For this review, take the finished solid that the model builds, in its own axes (mm). Face numbers are marked on the shaded views. Round coordinates to 2 decimals unless told otherwise and drop trailing zeros. Loops run counter-clockwise (first coordinate to the right, second up) from the corner with the lowest first, then second, coordinate; pieces in that order, holes last. Notation, with made-up numbers: M 18,0 L 49,0 A24 cw 49,31 Z; hole C 89,76.25 d8. An arc over 180 degrees is marked long. One line per question, with ' | ' between items. Start each with the question number.
1) We need section B-B (y = 0). Give the boundary of the cut face in (x, z).
2) For pin 1 Ø2.5 at (x, z) = (11, -0.5) entering from -Y (3 decimals); pin 2 Ø2 at (x, y) = (12, 9.5) entering from -Z; pin 3 Ø0.5 at (x, y) = (12.5, 5.5) entering from -Z, all flat-tipped, find the tip position at first contact; note any pin that passes through.
3) We need section A-A (z = 0). Give the boundary of the cut face in (x, y).
4) Mouldability with a two-part tool opening along Z and no side actions: class the marked faces 1, 2 and 3 as pulls with the +Z half, pulls with the -Z half, needs draft (parallel to the pull), parting line crosses it, or undercut.
5) For probe 1 along X at (y, z) = (-8.5, -6.75); probe 2 along Z at (x, y) = (14, 0); probe 3 along Z at (x, y) = (12.25, 9.25), list the stretches that pass through material, from the lowest coordinate up. Write a range as from..to.
```python
from build123d import *

# Parameters (mm, degrees)
SCHIZZO5_R                    = 0.75
TAGLIO_ESTRUSIONE1_DEPTH      = 7
TAGLIO_ESTRUSIONE2_REACH      = 26.782
TAGLIO_ESTRUSIONE2_END_RADIUS = 8
SCHIZZO6_R                    = 1.5
TAGLIO_ESTRUSIONE3_REACH      = 26.782
TAGLIO_ESTRUSIONE3_END_RADIUS = 8
SCHIZZO7_R                    = 1.5
SMUSSO1_SIZE                  = 0.5
SMUSSO2_SIZE                  = 0.25
SCHIZZO8_R                    = 5
TAGLIO_ESTRUSIONE4_DEPTH      = 25.781545622
TAGLIO_ESTRUSIONE5_START      = -7
SCHIZZO9_R                    = 8
TAGLIO_ESTRUSIONE5_DEPTH      = 7
TAGLIO_ESTRUSIONE6_DEPTH      = 30.654470544
TAGLIO_ESTRUSIONE6_DEPTH_BACK = 7
SCHIZZO10_W                   = 3
SCHIZZO10_H                   = 1.630303993


with BuildPart() as part:
    # Schizzo4 → Rivoluzione1 (revolve)
    with BuildSketch(Plane.XY, mode=Mode.PRIVATE) as rivoluzione1_sk:
        Polygon((0, 2.5), (0, 8), (7, 8), (7, 12.75), (7.75, 12.75), (8.5, 11.450961894), (8.5, 11.25), (15.5, 11.25), (15.5, 11.450961894), (16.25, 12.75), (17, 12.75), (17, 2.5), align=None)
    revolve(rivoluzione1_sk.sketch.rotate(Axis((0, 0, 0), (1, 0, 0)), 90), axis=Axis((0, 0, 0), (1, 0, 0)))

    # Schizzo5 → Taglio-Estrusione1 (cut)
    with BuildSketch(Plane(origin=(8.5, 0, 0), x_dir=(0, 0, -1), z_dir=(1, 0, 0))):
        with Locations((0, 11.25)):
            Circle(SCHIZZO5_R)
        with Locations((1.953541999, 11.079087221)):
            Circle(SCHIZZO5_R)
        with Locations((3.847726612, 10.571541984)):
            Circle(SCHIZZO5_R)
        with Locations((5.625, 9.742785793)):
            Circle(SCHIZZO5_R)
        with Locations((7.231360609, 8.617999985)):
            Circle(SCHIZZO5_R)
        with Locations((8.617999985, 7.231360609)):
            Circle(SCHIZZO5_R)
        with Locations((9.742785793, 5.625)):
            Circle(SCHIZZO5_R)
        with Locations((10.571541984, 3.847726612)):
            Circle(SCHIZZO5_R)
        with Locations((11.079087221, 1.953541999)):
            Circle(SCHIZZO5_R)
        with Locations((11.25, 0)):
            Circle(SCHIZZO5_R)
        with Locations((11.079087221, -1.953541999)):
            Circle(SCHIZZO5_R)
        with Locations((10.571541984, -3.847726612)):
            Circle(SCHIZZO5_R)
        with Locations((9.742785793, -5.625)):
            Circle(SCHIZZO5_R)
        with Locations((8.617999985, -7.231360609)):
            Circle(SCHIZZO5_R)
        with Locations((7.231360609, -8.617999985)):
            Circle(SCHIZZO5_R)
        with Locations((5.625, -9.742785793)):
            Circle(SCHIZZO5_R)
        with Locations((3.847726612, -10.571541984)):
            Circle(SCHIZZO5_R)
        with Locations((1.953541999, -11.079087221)):
            Circle(SCHIZZO5_R)
        with Locations((0, -11.25)):
            Circle(SCHIZZO5_R)
        with Locations((-1.953541999, -11.079087221)):
            Circle(SCHIZZO5_R)
        with Locations((-3.847726612, -10.571541984)):
            Circle(SCHIZZO5_R)
        with Locations((-5.625, -9.742785793)):
            Circle(SCHIZZO5_R)
        with Locations((-7.231360609, -8.617999985)):
            Circle(SCHIZZO5_R)
        with Locations((-8.617999985, -7.231360609)):
            Circle(SCHIZZO5_R)
        with Locations((-9.742785793, -5.625)):
            Circle(SCHIZZO5_R)
        with Locations((-10.571541984, -3.847726612)):
            Circle(SCHIZZO5_R)
        with Locations((-11.079087221, -1.953541999)):
            Circle(SCHIZZO5_R)
        with Locations((-11.25, 0)):
            Circle(SCHIZZO5_R)
        with Locations((-11.079087221, 1.953541999)):
            Circle(SCHIZZO5_R)
        with Locations((-10.571541984, 3.847726612)):
            Circle(SCHIZZO5_R)
        with Locations((-9.742785793, 5.625)):
            Circle(SCHIZZO5_R)
        with Locations((-8.617999985, 7.231360609)):
            Circle(SCHIZZO5_R)
        with Locations((-7.231360609, 8.617999985)):
            Circle(SCHIZZO5_R)
        with Locations((-5.625, 9.742785793)):
            Circle(SCHIZZO5_R)
        with Locations((-3.847726612, 10.571541984)):
            Circle(SCHIZZO5_R)
        with Locations((-1.953541999, 11.079087221)):
            Circle(SCHIZZO5_R)
    extrude(amount=TAGLIO_ESTRUSIONE1_DEPTH, mode=Mode.SUBTRACT)

    # Taglio-Estrusione2: up to this cylinder (the profile starts inside it)
    taglio_estrusione2_end = Plane(origin=(3.5, 0, 0), z_dir=(-1, 0, 0)) * Cylinder(TAGLIO_ESTRUSIONE2_END_RADIUS, 70.564, mode=Mode.PRIVATE)
    # Schizzo6 → Taglio-Estrusione2 (cut, up to the surface)
    with BuildSketch(Plane.XY, mode=Mode.PRIVATE) as taglio_estrusione2_sk1:
        with Locations(Location((3.5, 0, 0), (0, 0, 180))):
            Circle(SCHIZZO6_R)
    taglio_estrusione2_tool1 = extrude(taglio_estrusione2_sk1.sketch, amount=TAGLIO_ESTRUSIONE2_REACH, mode=Mode.PRIVATE) & taglio_estrusione2_end
    add(taglio_estrusione2_tool1.solids().sort_by_distance((3.5, 0, 0))[0], mode=Mode.SUBTRACT)

    # Taglio-Estrusione3: up to this cylinder (the profile starts inside it)
    taglio_estrusione3_end = Plane(origin=(3.5, 0, 0), z_dir=(-1, 0, 0)) * Cylinder(TAGLIO_ESTRUSIONE3_END_RADIUS, 70.564, mode=Mode.PRIVATE)
    # Schizzo7 → Taglio-Estrusione3 (cut, up to the surface)
    with BuildSketch(Plane(origin=(0, 0, 0), x_dir=(1, 0, 0), z_dir=(0, 1, 0)), mode=Mode.PRIVATE) as taglio_estrusione3_sk1:
        with Locations(Location((3.5, 0, 0), (0, 0, 90))):
            Circle(SCHIZZO7_R)
    taglio_estrusione3_tool1 = extrude(taglio_estrusione3_sk1.sketch, amount=TAGLIO_ESTRUSIONE3_REACH, mode=Mode.PRIVATE) & taglio_estrusione3_end
    add(taglio_estrusione3_tool1.solids().sort_by_distance((3.5, 0, 0))[0], mode=Mode.SUBTRACT)

    # Smusso1
    smusso1_edges = [part.edges().sort_by_distance(p)[0] for p in [
        (0, 0, -8),
        (0, 0, -2.5),
    ]]
    chamfer(smusso1_edges, length=SMUSSO1_SIZE)

    # Smusso2
    smusso2_edges = [part.edges().sort_by_distance(p)[0] for p in [
        (7, 0, -12.75),
        (17, 0, -12.75),
    ]]
    chamfer(smusso2_edges, length=SMUSSO2_SIZE)

    # Schizzo8 → Taglio-Estrusione4 (cut, through all)
    with BuildSketch(Plane.ZY):
        Circle(SCHIZZO8_R)
    extrude(amount=-TAGLIO_ESTRUSIONE4_DEPTH, mode=Mode.SUBTRACT)

    # Schizzo9 → Taglio-Estrusione5 (cut)
    with BuildSketch(Plane.ZY.offset(TAGLIO_ESTRUSIONE5_START)):
        Circle(SCHIZZO9_R)
    extrude(amount=TAGLIO_ESTRUSIONE5_DEPTH, mode=Mode.SUBTRACT)

    # Schizzo10 → Taglio-Estrusione6 (cut, two sides: drawn at the far end of the back side and taken through both)
    with BuildSketch(Plane(origin=(15.5, 3.134798291, -10.804422228), x_dir=(0, 0, 1), z_dir=(-1, 0, 0)).offset(-TAGLIO_ESTRUSIONE6_DEPTH_BACK)):
        with Locations((10.804422228, 2.450049713)):
            Rectangle(SCHIZZO10_W, SCHIZZO10_H)
    extrude(amount=TAGLIO_ESTRUSIONE6_DEPTH + TAGLIO_ESTRUSIONE6_DEPTH_BACK, mode=Mode.SUBTRACT)


solid = part.part
```
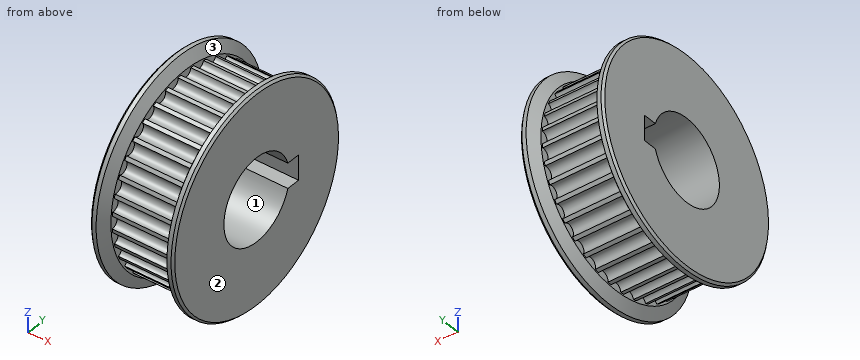
Answers below:
1) outline: M 7,-12.5 L 7.25,-12.75 L 7.75,-12.75 L 8.5,-11.45 L 8.5,-10.5 L 15.5,-10.5 L 15.5,-11.45 L 16.25,-12.75 L 16.75,-12.75 L 17,-12.5 L 17,-5 L 7,-5 Z; M 7,5 L 17,5 L 17,12.5 L 16.75,12.75 L 16.25,12.75 L 15.5,11.45 L 15.5,10.5 L 8.5,10.5 L 8.5,11.45 L 7.75,12.75 L 7.25,12.75 L 7,12.5 Z
2) pin 1: y = -11.225 | pin 2: z = -6.64 | pin 3: z = -9.09
3) outline: M 7,-12.5 L 7.25,-12.75 L 7.75,-12.75 L 8.5,-11.45 L 8.5,-10.5 L 15.5,-10.5 L 15.5,-11.45 L 16.25,-12.75 L 16.75,-12.75 L 17,-12.5 L 17,-5 L 7,-5 Z; M 7,6.4 L 17,6.4 L 17,12.5 L 16.75,12.75 L 16.25,12.75 L 15.5,11.45 L 15.5,10.5 L 8.5,10.5 L 8.5,11.45 L 7.75,12.75 L 7.25,12.75 L 7,12.5 Z
4) face 1: undercut | face 2: needs draft | face 3: parting line crosses it
5) probe 1: 7..8.5, 15.5..17 | probe 2: -10.5..-5, 5..10.5 | probe 3: -6.4..-6.19, -5.06..5.06, 6.19..6.4
